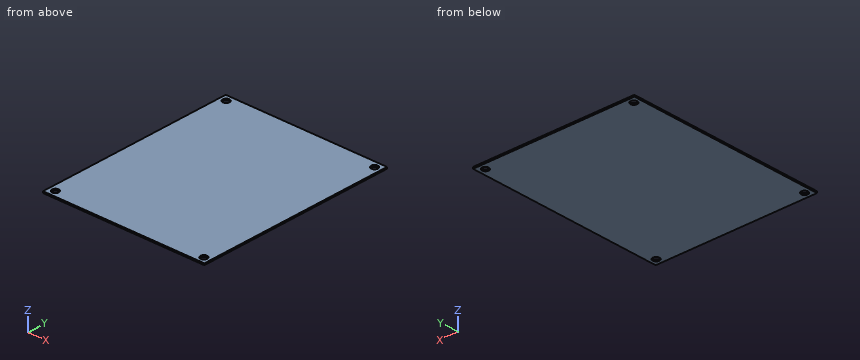
from build123d import *

# Parameters (mm, degrees)
F0_W     = 100
F0_H     = 123
F1_DEPTH = 1
F2_D     = 4.2
F2_DEPTH = 7


with BuildPart() as f1:
    # F0 (on Top) → F1 (new body)
    with BuildSketch(Plane.XY):
        Rectangle(F0_W, F0_H)
    extrude(amount=-F1_DEPTH)

    # F2
    with Locations(Plane.XY):
        with Locations((-46, 57.5), (-46, -57.5), (46, -57.5), (46, 57.5)):
            Hole(F2_D / 2, depth=F2_DEPTH)


solid = f1.part
Part model, mm, in its own coordinate system. Coordinates: 2 decimals unless noted, no trailing zeros. Loops run counter-clockwise (first coordinate to the right, second up) from the corner with the lowest first, then second, coordinate; pieces in that order, holes last. Notation, with made-up numbers: M 84,51.5 L 98,51.5 A12 ccw 98,59.5 Z; hole C 21,-13.5 d8. An arc over 180 degrees is marked long. Use a Markdown table: item, result. Add a question column.
Q1. Cut at B-B (x = -46). Write the cut outline in (y, z), and give its area (3 significant figures).
Q2. Pin check, flat tip, straight feed: P1, Ø6.5, axis at x = -46, y = -57.5, coming from the +Z side. Stop position of the tip, or through.
Q3. Cut at A-A (y = -57.5). Write the cut outline in (x, z), and give its area (3 significant figures).
Q4. Probe L1, parallel to Y at x = 46, z = -0.65. List the from-to ranges inside material, lowest first.
Worked out:
| question | item | result |
|---|---|---|
| 1 | outline | M -61.5,-1 L -59.6,-1 L -59.6,0 L -61.5,0 Z; M -55.4,-1 L 55.4,-1 L 55.4,0 L -55.4,0 Z; M 59.6,-1 L 61.5,-1 L 61.5,0 L 59.6,0 Z |
| 1 | area | 115 mm2 |
| 2 | P1 | stops at z = 0 |
| 3 | outline | M -50,-1 L -48.1,-1 L -48.1,0 L -50,0 Z; M -43.9,-1 L 43.9,-1 L 43.9,0 L -43.9,0 Z; M 48.1,-1 L 50,-1 L 50,0 L 48.1,0 Z |
| 3 | area | 91.6 mm2 |
| 4 | L1 | y = -61.5 to -59.6, -55.4 to 55.4, 59.6 to 61.5 |
